Design review of the part built by this model. Coordinates are the model's own, in mm. A direction names the side the tool comes from. Coordinates: 2 decimals unless noted, no trailing zeros. Loops run counter-clockwise (first coordinate to the right, second up) from the corner with the lowest first, then second, coordinate; pieces in that order, holes last. Notation, with made-up numbers: (49.25, 54) -> (70.25, 54) arc R26 ccw to (70.25, 88) -> close; hole circle Ø6 at (-33.75, -17.5). An arc over 180 degrees is marked (long way). Use CSV: the item, a comma, the result in double quotes.
```python
from build123d import *

# Parameters (mm, degrees)
BOSS_EXTRU_1_DEPTH      = 50
BOSS_EXTRU_2_START      = 50
BOSS_EXTRU_2_DEPTH      = 4
ESQUISSE3_R             = 1.5
ENL_V_MAT_EXTRU_1_DEPTH = 82.186513658
ESQUISSE4_W             = 14
ESQUISSE4_H             = 17
ESQUISSE4_W_2           = 16
ESQUISSE4_H_2           = 16
ESQUISSE4_W_3           = 6
ESQUISSE4_H_3           = 10
ENL_V_MAT_EXTRU_4_DEPTH = 4
ESQUISSE5_W             = 50
ESQUISSE5_H             = 3
ENL_V_MAT_EXTRU_5_DEPTH = 4


with BuildPart() as part:
    # Esquisse1 → Boss.-Extru.1 (new body)
    with BuildSketch(Plane.XY):
        with BuildLine():
            Line((-46.5, -35), (46.5, -35))
            ThreePointArc((46.5, -35), (48.621320344, -34.121320344), (49.5, -32))
            Line((49.5, -32), (49.5, 32))
            ThreePointArc((49.5, 32), (48.621320344, 34.121320344), (46.5, 35))
            Line((46.5, 35), (-46.5, 35))
            ThreePointArc((-46.5, 35), (-48.621320344, 34.121320344), (-49.5, 32))
            Line((-49.5, 32), (-49.5, -32))
            ThreePointArc((-49.5, -32), (-48.621320344, -34.121320344), (-46.5, -35))
        make_face()
        with BuildLine():
            ThreePointArc((44.5, -33), (46.621320344, -32.121320344), (47.5, -30))
            Line((47.5, -30), (47.5, 30))
            ThreePointArc((47.5, 30), (46.621320344, 32.121320344), (44.5, 33))
            Line((44.5, 33), (-44.5, 33))
            ThreePointArc((-44.5, 33), (-46.621320344, 32.121320344), (-47.5, 30))
            Line((-47.5, 30), (-47.5, -30))
            ThreePointArc((-47.5, -30), (-46.621320344, -32.121320344), (-44.5, -33))
            Line((-44.5, -33), (44.5, -33))
        make_face(mode=Mode.SUBTRACT)
    extrude(amount=BOSS_EXTRU_1_DEPTH)

    # Esquisse2 → Boss.-Extru.2 (add)
    with BuildSketch(Plane.XY.offset(BOSS_EXTRU_2_START)):
        with BuildLine():
            Line((-46.5, -35), (46.5, -35))
            ThreePointArc((46.5, -35), (48.621320344, -34.121320344), (49.5, -32))
            Line((49.5, -32), (49.5, 32))
            ThreePointArc((49.5, 32), (48.621320344, 34.121320344), (46.5, 35))
            Line((46.5, 35), (-46.5, 35))
            ThreePointArc((-46.5, 35), (-48.621320344, 34.121320344), (-49.5, 32))
            Line((-49.5, 32), (-49.5, -32))
            ThreePointArc((-49.5, -32), (-48.621320344, -34.121320344), (-46.5, -35))
        make_face()
    extrude(amount=BOSS_EXTRU_2_DEPTH)

    # Esquisse3 → Enlèv. mat.-Extru.1 (cut, through all)
    with BuildSketch(Plane.XY.offset(54)):
        with Locations((39.5, 24.5)):
            Circle(ESQUISSE3_R)
        with Locations((-18.5, 24.5)):
            Circle(ESQUISSE3_R)
        with Locations((39.5, -24.5)):
            Circle(ESQUISSE3_R)
        with Locations((-18.5, -24.5)):
            Circle(ESQUISSE3_R)
    extrude(amount=-ENL_V_MAT_EXTRU_1_DEPTH, mode=Mode.SUBTRACT)

    # Esquisse4 → Enlèv. mat.-Extru.4 (cut)
    with BuildSketch(Plane(origin=(-49.5, 0, 0), x_dir=(0, 0, -1), z_dir=(1, 0, 0))):
        with Locations((-37.5, -18)):
            Rectangle(ESQUISSE4_W, ESQUISSE4_H)
        with Locations((-36, 1)):
            Rectangle(ESQUISSE4_W_2, ESQUISSE4_H_2)
        with Locations((-36, 19)):
            Rectangle(ESQUISSE4_W_2, ESQUISSE4_H_2)
        with Locations((-13, 0)):
            Rectangle(ESQUISSE4_W_3, ESQUISSE4_H_3)
    extrude(amount=ENL_V_MAT_EXTRU_4_DEPTH, mode=Mode.SUBTRACT)

    # Esquisse5 → Enlèv. mat.-Extru.5 (cut)
    with BuildSketch(Plane(origin=(0, 35, 0), x_dir=(1, 0, 0), z_dir=(0, 1, 0))):
        with Locations((0, -27.5)):
            Rectangle(ESQUISSE5_W, ESQUISSE5_H)
    extrude(amount=-ENL_V_MAT_EXTRU_5_DEPTH, mode=Mode.SUBTRACT)


solid = part.part
```
Item 1: Draft analysis for pull direction X (two halves, no side actions). For faces 1 (the face through (-47.5, 0, 19)), 2 (the face through (-49.5, 0, 27)), 3 (the face through (-15, -34, 0)), state which applies: pulls with the +X half, pulls with the -X half, needs draft (parallel to the pull), parting line crosses it, or undercut.
Checked values:
face 1,"undercut"
face 2,"pulls with the -X half"
face 3,"needs draft"
Item 2: Clearance check with flat-ended pins moving along their axes: pin 1 (2 mm diameter, centred on x = -49, z = 37.5, fed in from +Y); pin 2 (1.6 mm diameter, centred on y = 34, z = 27.5, fed in from +X); pin 3 (1.6 mm diameter, centred on x = -48.5, y = 1, fed in from -Z); pin 4 (1 mm diameter, centred on x = -48.5, z = 38.5, fed in from -Y). State where each tip first meets the part, or that it passes through.
Checked values:
pin 1,"y = 34.6"
pin 2,"x = 49.25"
pin 3,"z = 0"
pin 4,"y = -34.6"
Item 3: Add section C-C (x = 39.5). Give the boundary of the cut face in (y, z).
Checked values:
outline,"(-35, 0) -> (-33, 0) -> (-33, 50) -> (-26, 50) -> (-26, 54) -> (-35, 54) -> close; (-23, 50) -> (23, 50) -> (23, 54) -> (-23, 54) -> close; (26, 50) -> (33, 50) -> (33, 0) -> (35, 0) -> (35, 54) -> (26, 54) -> close"
Item 4: Machinability: for faces 4 (the face through (-49, 1, 44)), 5 (the face through (-25, 34, 28)), 6 (the face through (47.5, 0, 25)), which of the approach directions +Z, -Z, +X, -X, +Y, -Y give a long, thin tool a straight path to every point of the face, cutting with its end or side? Answer none if there is none.
Checked values:
face 4,"-X"
face 5,"+Y"
face 6,"-Z"
Item 5: Add section B-B (y = -24.5). Give the boundary of the cut face in (x, z), then the cut area to 3 significant figures.
Checked values:
outline,"(-49.5, 0) -> (-47.5, 0) -> (-47.5, 30.5) -> (-49.5, 30.5) -> close; (-49.5, 44.5) -> (-47.5, 44.5) -> (-47.5, 50) -> (-20, 50) -> (-20, 54) -> (-49.5, 54) -> close; (-17, 50) -> (38, 50) -> (38, 54) -> (-17, 54) -> close; (41, 50) -> (47.5, 50) -> (47.5, 0) -> (49.5, 0) -> (49.5, 54) -> (41, 54) -> close"
area,"544 mm^2"
Item 6: Add section D-D (y = -13.5). Give the boundary of the cut face in (x, z), then the cut area to 3 significant figures.
Checked values:
outline,"(-49.5, 0) -> (-47.5, 0) -> (-47.5, 30.5) -> (-49.5, 30.5) -> close; (-49.5, 44.5) -> (-47.5, 44.5) -> (-47.5, 50) -> (47.5, 50) -> (47.5, 0) -> (49.5, 0) -> (49.5, 54) -> (-49.5, 54) -> close"
area,"568 mm^2"
Item 7: Add section A-A (x = -18.5). Give the boundary of the cut face in (y, z), then the cut area to 3 significant figures.
Checked values:
outline,"(-35, 0) -> (-33, 0) -> (-33, 50) -> (-26, 50) -> (-26, 54) -> (-35, 54) -> close; (-23, 50) -> (23, 50) -> (23, 54) -> (-23, 54) -> close; (26, 50) -> (33, 50) -> (33, 29) -> (35, 29) -> (35, 54) -> (26, 54) -> close; (33, 0) -> (35, 0) -> (35, 26) -> (33, 26) -> close"
area,"450 mm^2"
Item 8: To check wall thickness, follow line 1 along Y through (x, z) = (-18.5, 51); line 2 along X through (y, z) = (25, 26.5); line 3 along Y through (x, z) = (37, 40). State the ranges of each line that lie inside material, in increasing order.
Checked values:
line 1,"-35 to -26, -23 to 23, 26 to 35"
line 2,"-49.5 to -47.5, 47.5 to 49.5"
line 3,"-35 to -33, 33 to 35"
